Autodesk Inventor part; units mm, degrees
ref_plane "YZ Plane" through (0, 0, 0) normal (1, 0, 0) x (0, 1, 0)
ref_plane "XZ Plane" through (0, 0, 0) normal (0, 1, 0) x (-1, 0, 0)
ref_plane "XY Plane" through (0, 0, 0) normal (0, 0, 1) x (1, 0, 0)
sketch "Sketch1" plane through (0, 0, 0) normal (0, 0, 1) x (1, 0, 0)
  arc A0 (-5.6835, 2.2943) -> (-7.6273, -2.3122) centre (-6.6766, 0) ccw
  arc A1 (-5.2258, 2.1583) -> (0.2129, 2.4842) centre (-3.2055, 13.987) ccw
  line L0 (-6.6766, 2.5) -> (-6.6766, -2.5) construction
  arc A2 (-5.6835, 2.2943) -> (-5.2258, 2.1583) centre (-4.8891, 4.1298) ccw
  arc A3 (1.5395, -2.4196) -> (1.4069, 2.4672) centre (0.5964, 0) ccw
  arc A4 (1.4069, 2.4672) -> (0.2129, 2.4842) centre (0.7827, 0.5671) ccw
  line L1 (0.5964, 2.5969) -> (0.5964, -2.5969) construction
  arc A5 (0.1965, -2.4587) -> (-6.2967, -2.3795) centre (-3.1776, -12.8694) ccw
  arc A6 (-7.6273, -2.3122) -> (-6.2967, -2.3795) centre (-6.8667, -0.4624) ccw
  arc A7 (0.1965, -2.4587) -> (1.5395, -2.4196) centre (0.8132, -0.5562) ccw
  circle A8 centre (-6.6766, 0) radius 1
  circle A9 centre (0.5964, 0) radius 1.5
  line L2 (1.4069, 2.4672) -> (2.7069, 4.2755)
  line L3 (3.1306, 0.5671) -> (4.6306, 2.3807)
  arc A10 (4.6306, 2.3807) -> (2.7069, 4.2755) centre (1.4088, 1.0336) ccw
  line L4 (-3.2055, 1.987) -> (-3.2055, -1.9256) construction
  line L5 (-3.2055, 1.987) -> (-3.2055, -1.9256) construction
  arc A11 (-3.2055, -1.9256) -> (-3.2055, 1.987) centre (-7.3367, 0.0307) ccw
  point P0 (0, 0)
  dimension "d0" = 5
  dimension "d1" = 12
  dimension "d2" = 2
  dimension "d3" = 2
  dimension "d5" = 2
  dimension "d6" = 2
  dimension "d7" = 3
  dimension "d8" = 1.5
  dimension "d9" = 1.3
extrude "Extrusion1" add sketch "Sketch1" along normal blind 1 contours A2 A1 A11 A5 A6 A0
extrude "Extrusion2" add sketch "Sketch1" against normal blind 1 contours A1 A4 A3 A7 A5 A11
extrude "Extrusion3" add sketch "Sketch1" against normal blind 1 contours L2 A10 L3 A3
sketch "Esboço2" plane through (0, 0, 0) normal (0, 0, -1) x (-1, 0, 0)
  line L0 (4.0311, 2.0155) -> (4.0311, -1.9589)
  arc A0 (3.2055, 1.987) -> (3.2055, -1.9256) centre (7.3367, 0.0307) ccw
  arc A1 (3.2055, 1.987) -> (3.2055, -1.9256) centre (7.3367, 0.0307) ccw
  arc A2 (3.2055, 1.987) -> (5.2258, 2.1583) centre (3.2055, 13.987) ccw
  arc A3 (6.2967, -2.3795) -> (3.2055, -1.9256) centre (3.1776, -12.8694) ccw
  point P0 (0, 0)
extrude "Extrusão4" add sketch "Esboço2" along normal blind 1
fillet "Arredondamento1" radius 0.7 1 edges at (-4.0311, 0.0283, -1)
properties material "Nickel-Copper Alloy 400"
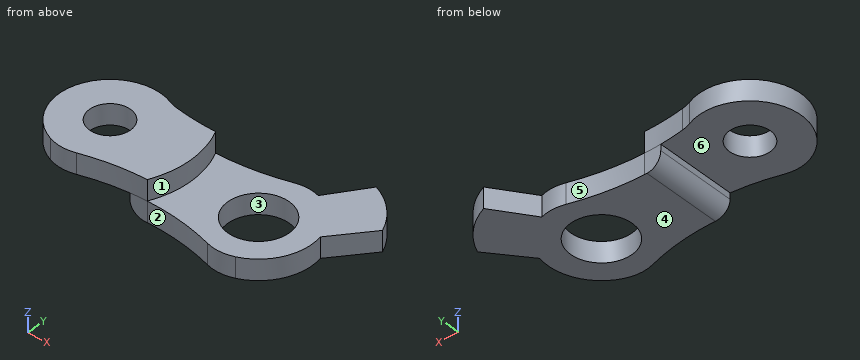
Geometry check sheet. Reference: the model listing, model coordinates, mm. Face numbers are marked on the shaded views. A direction names the side the tool comes from. Coordinates: 2 decimals unless noted, no trailing zeros. Write each loop counter-clockwise with the first axis right and the second up, starting at its lowest first coordinate (ties: lowest second). Pieces come first, ordered by that corner, then holes. Notation, with made-up numbers: (-3, 77.25) -> (23, 77.25) arc R20 cw to (23, 95.25) -> close; hole circle Ø7 at (-9.5, -5.75). An arc over 180 degrees is marked (long way). Use CSV: the item, a comma, the result in double quotes. Start each with the question number.
Item 1: Cross-section at B-B, the plane y = 0. Record the cut outline in (x, z).
Item 2: Set-up check for the marked faces 4, 5 and 6: record each of +Z, -Z, +X, -X, +Y, -Y from which the full face is reachable in a straight line by a thin tool's end or side.
Item 3: Mould release check, pull along Y, two halves, no side actions. Record for the marked faces 1, 2 and 3: released by +Y, released by -Y, zero draft, split by the parting line, or undercut.
Item 4: Cross-section at D-D, the plane x = -6.75. Record the cut outline in (y, z), plus the area to 3 significant figures.
Item 5: Cross-section at A-A, the plane y = 1.25. Record the cut outline in (x, z), plus the area to 3 significant figures.
Item 6: Depth check by flat-ended pin: pin 1 Ø3.5 at (x, y) = (0.6, 0) entering from +Z; pin 2 Ø4 at (x, y) = (-6.5, 1) entering from -Z. Enter the tip coordinate at first touch or a pass-through.
Item 7: Thickness scan on line 1 (Z direction, x = -1, y = 1.5); line 2 (Z direction, x = -6.75, y = -2); line 3 (X direction, y = -0.25, z = -0.15). Record the ranges inside material, lowest first.
Item 8: Cross-section at C-C, the plane x = 1.25. Record the cut outline in (y, z), plus the area to 3 significant figures.
Answers:
1,outline,"(-9.18, 0) -> (-7.68, 0) -> (-7.68, 1) -> (-9.18, 1) -> close; (-5.68, 0) -> (-4.03, 0) -> (-4.03, -0.3) arc R0.7 ccw to (-3.33, -1) -> (-0.9, -1) -> (-0.9, 0) -> (-2.77, 0) -> (-2.77, 1) -> (-5.68, 1) -> close; (2.1, -1) -> (3.19, -1) -> (3.19, 0) -> (2.1, 0) -> close"
2,face 4,"-Z, +X, -X, +Y, -Y"
2,face 5,"+Z, -Z, +Y"
2,face 6,"-Z, -X, +Y, -Y"
3,face 1,"split by the parting line"
3,face 2,"released by -Y"
3,face 3,"undercut"
4,outline,"(-2.46, 0) -> (-1, 0) -> (-1, 1) -> (-2.46, 1) -> close; (1, 0) -> (2.5, 0) -> (2.5, 1) -> (1, 1) -> close"
4,area,"2.96 mm^2"
5,outline,"(-8.84, 0) -> (-4.03, 0) -> (-4.03, -0.3) arc R0.7 ccw to (-3.33, -1) -> (-0.23, -1) -> (-0.23, 0) -> (-2.93, 0) -> (-2.93, 1) -> (-8.84, 1) -> close; (1.43, -1) -> (3.7, -1) -> (3.7, 0) -> (1.43, 0) -> close"
5,area,"11.9 mm^2"
6,pin 1,"z = 0"
6,pin 2,"z = 0"
7,line 1,"-1 to 0"
7,line 2,"0 to 1"
7,line 3,"-4.03 to -0.88, 2.08 to 3.18"
8,outline,"(-2.51, -1) -> (-1.35, -1) -> (-1.35, 0) -> (-2.51, 0) -> close; (1.35, -1) -> (2.51, -1) -> (2.51, 0) -> (1.35, 0) -> close"
8,area,"2.32 mm^2"
